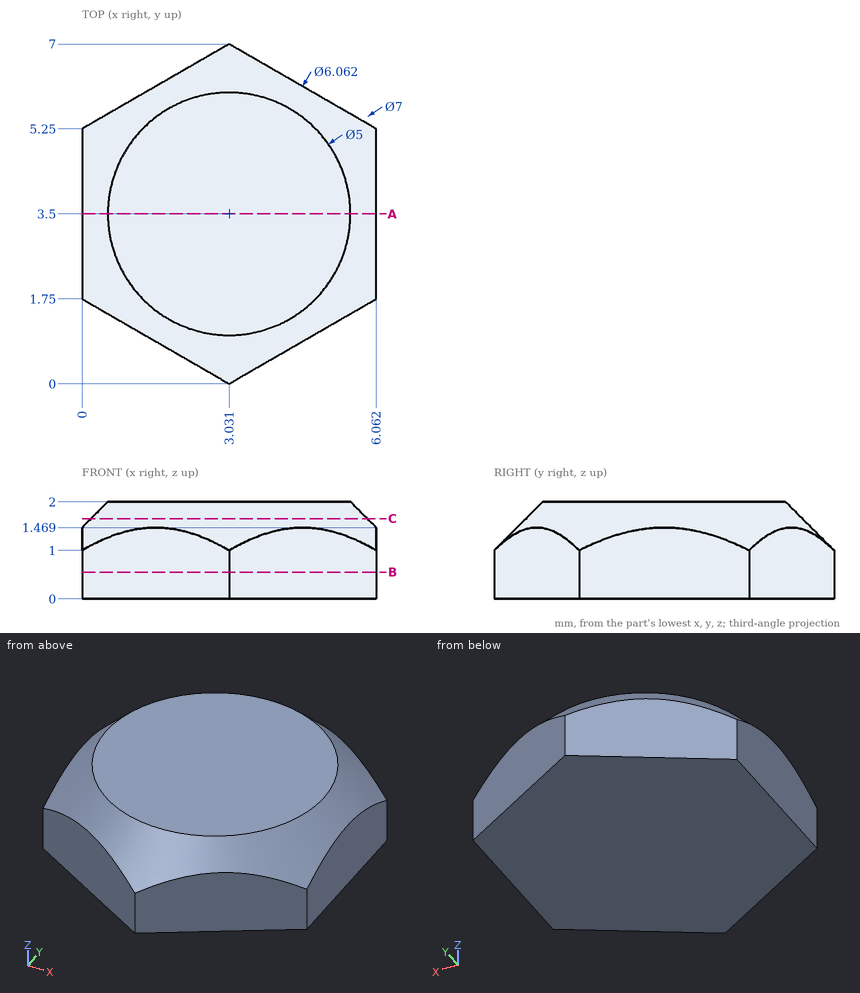
Verification items for this drawing (mm, ordinates from the low corner). Give positions to 0.01 mm unless a question says otherwise; leave off trailing zeros. Loops run counter-clockwise (first coordinate to the right, second up) from the corner with the lowest first, then second, coordinate; pieces in that order, holes last. Notation, with made-up numbers: M 69,-40 L 84,-40 A7 ccw 84,-36 Z; hole C -4,75.5 d3. An arc over 180 degrees is marked long. Answer as a JSON object with one key per item and string values. Group by question number.
Q1. Cross-section at C-C on z = 1.65. Record the cut outline in (x, y).
Q2. Material ranges on line 1 along Y through (x, z) = (4.5, 0.7); line 2 along X through (y, z) = (6.5, 0.7) (1 decimal); line 3 along Y through (x, z) = (4.75, 1), recorded low to high. Write a range as [from, to].
Q3. Cross-section at A-A on y = 3.5. Record the cut outline in (x, z), then the cut area to 3 significant figures.
Q4. Cross-section at B-B on z = 0.55. Record the cut outline in (x, y).
Evaluation:
{
 "1": {"outline": "C 3.03,3.5 d5.7"},
 "2": {"line 1": "y = [0.85, 6.15]", "line 2": "x = [2.2, 3.9]", "line 3": "y = [0.99, 6.01]"},
 "3": {"outline": "M 0,0 L 6.06,0 L 6.06,1.47 L 5.53,2 L 0.53,2 L 0,1.47 Z", "area": "11.8 mm2"},
 "4": {"outline": "M 0,1.75 L 3.03,0 L 6.06,1.75 L 6.06,5.25 L 3.03,7 L 0,5.25 Z"}
}
